Design review of the part shown in the three views and the two pictorial views. Dimensions are in mm from the part's minimum x, y and z. Coordinates: 2 decimals unless noted, no trailing zeros. Write each loop counter-clockwise with the first axis right and the second up, starting at its lowest first coordinate (ties: lowest second). Pieces come first, ordered by that corner, then holes. Notation, with made-up numbers: (18, 36) - (42, 36) arc R25 cw to (42, 70) - close; hole circle Ø6 at (-12, 84). An arc over 180 degrees is marked (long way). Return JSON: item names as keys, results as strings. Group by question number.
(1) We need section B-B on y = 14.5. State the section outline as (x, z) points.
(2) For pin 1 Ø4 at (x, y) = (13.5, 19) entering from +Z; pin 2 Ø2 at (x, y) = (49.5, 50.5) entering from +Z; pin 3 Ø0.9 at (x, z) = (31.5, 4.5) entering from +Y, all flat-tipped, find the tip position at first contact; note any pin that passes through.
(3) To check wall thickness, follow L1, parallel to Y at x = 9.68, z = 7.5; L2, parallel to X at y = 56, z = 4.75; L3, parallel to X at y = 9, z = 6.75. State the ranges of each line that lie inside material, in increasing order. Write a range as from..to.
(4) Draft analysis for pull direction X (two halves, no side actions). For the marked faces 1 and 2, state which applies: released by +X, released by -X, zero draft, split by the parting line, or undercut.
(5) We need section A-A on z = 9.25. State the section outline as (x, y) points, then the cut area to 3 significant figures.
(6) We need section C-C on x = 50.32. State the section outline as (y, z) points.
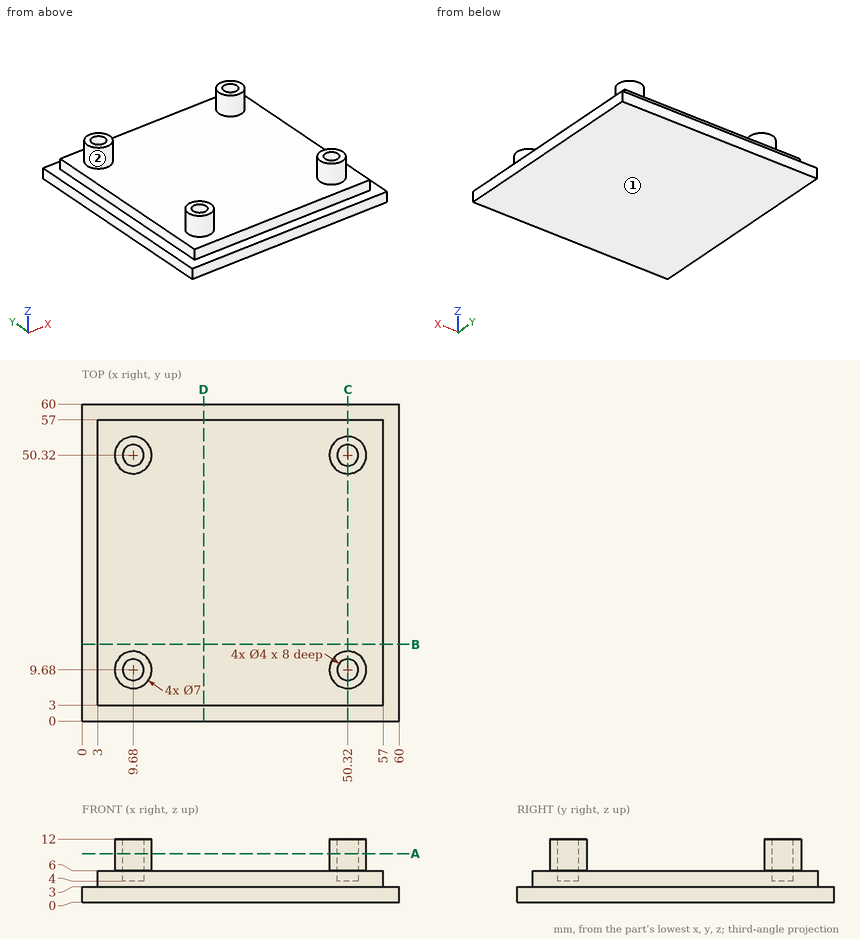
Ans:
{
 "1": {"outline": "(0, 0) - (60, 0) - (60, 3) - (57, 3) - (57, 6) - (3, 6) - (3, 3) - (0, 3) - close"},
 "2": {"pin 1": "z = 6", "pin 2": "z = 4", "pin 3": "y = 57"},
 "3": {"L1": "6.18..7.68, 11.68..13.18, 46.82..48.32, 52.32..53.82", "L2": "3..57", "L3": "6.25..7.8, 11.56..13.11, 46.89..48.44, 52.2..53.75"},
 "4": {"face 1": "zero draft", "face 2": "undercut"},
 "5": {"outline": "circle Ø7 at (9.68, 9.68); circle Ø7 at (9.68, 50.32); circle Ø7 at (50.32, 9.68); circle Ø7 at (50.32, 50.32); hole circle Ø4 at (9.68, 9.68); hole circle Ø4 at (9.68, 50.32); hole circle Ø4 at (50.32, 9.68); hole circle Ø4 at (50.32, 50.32)", "area": "104 mm²"},
 "6": {"outline": "(0, 0) - (60, 0) - (60, 3) - (57, 3) - (57, 6) - (53.82, 6) - (53.82, 12) - (52.32, 12) - (52.32, 4) - (48.32, 4) - (48.32, 12) - (46.82, 12) - (46.82, 6) - (13.18, 6) - (13.18, 12) - (11.68, 12) - (11.68, 4) - (7.68, 4) - (7.68, 12) - (6.18, 12) - (6.18, 6) - (3, 6) - (3, 3) - (0, 3) - close"}
}
